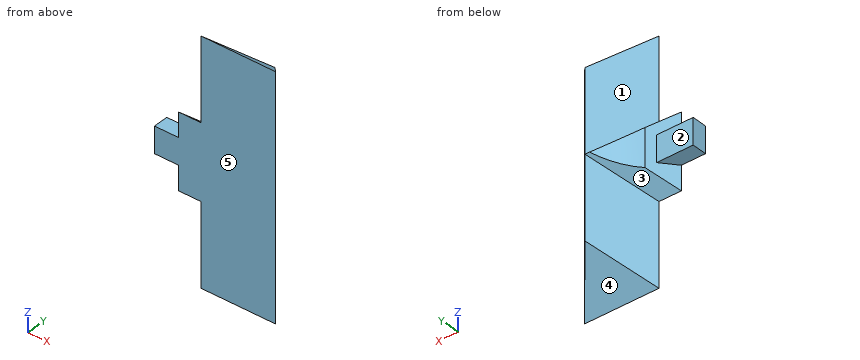
from build123d import *

# Parameters (mm, degrees)
BOSS_EXTRUDE1_START       = -105
BOSS_EXTRUDE1_DEPTH       = 160
BOSS_EXTRUDE1_2_DEPTH     = 40
BOSS_EXTRUDE1_START_2     = -20
BOSS_EXTRUDE1_3_OUTLINE_W = 47
BOSS_EXTRUDE1_3_OUTLINE_H = 147
BOSS_EXTRUDE1_3_DEPTH     = 20
BOSS_EXTRUDE1_START_3     = 42.132444372
BOSS_EXTRUDE1_4_OUTLINE_W = 53
BOSS_EXTRUDE1_4_OUTLINE_H = 116
BOSS_EXTRUDE1_4_DEPTH     = 19.867555628
BOSS_EXTRUDE1_START_4     = 80.434666527
BOSS_EXTRUDE1_5_OUTLINE_W = 52
BOSS_EXTRUDE1_5_OUTLINE_H = 117
BOSS_EXTRUDE1_5_DEPTH     = 20.565333473
SKETCH2_W                 = 32.400830654
SKETCH2_H                 = 17.550449938
BOSS_EXTRUDE2_DEPTH       = 10
SKETCH4_R                 = 75
CUT_EXTRUDE1_DEPTH        = 80


with BuildPart() as part:
    # Boss-Extrude1: read off the stored shape, not the designer's step
    # Boss-Extrude1 outline → Boss-Extrude1 (new body)
    with BuildSketch(Plane.XY.offset(BOSS_EXTRUDE1_START)):
        Polygon((65, 0), (40, 29.793839815), (15, 0), align=None)
    extrude(amount=BOSS_EXTRUDE1_DEPTH)

    # Boss-Extrude1 2 outline → Boss-Extrude1 2 (add)
    with BuildSketch(Plane.YZ):
        Polygon((0, -50), (29.793839815, -25), (0, 0), align=None)
    extrude(amount=BOSS_EXTRUDE1_2_DEPTH)

    # Boss-Extrude1 3 outline → Boss-Extrude1 3 (cut)
    with BuildSketch(Plane(origin=(0, 0, 0), x_dir=(0.6427876096865404, 0.7660444431189772, 0), z_dir=(0.7660444431189772, -0.6427876096865403, 0)).offset(BOSS_EXTRUDE1_START_2)):
        with Locations((22.5, -24.5)):
            Rectangle(BOSS_EXTRUDE1_3_OUTLINE_W, BOSS_EXTRUDE1_3_OUTLINE_H)
    extrude(amount=BOSS_EXTRUDE1_3_DEPTH, mode=Mode.SUBTRACT)

    # Boss-Extrude1 4 outline → Boss-Extrude1 4 (cut)
    with BuildSketch(Plane(origin=(0, 0, 0), x_dir=(1, 0, 0), z_dir=(0, 0.6427876096865403, 0.7660444431189772)).offset(BOSS_EXTRUDE1_START_3)):
        with Locations((40.5, 21)):
            Rectangle(BOSS_EXTRUDE1_4_OUTLINE_W, BOSS_EXTRUDE1_4_OUTLINE_H)
    extrude(amount=BOSS_EXTRUDE1_4_DEPTH, mode=Mode.SUBTRACT)

    # Boss-Extrude1 5 outline → Boss-Extrude1 5 (cut)
    with BuildSketch(Plane(origin=(0, 0, 0), x_dir=(1, 0, 0), z_dir=(0, 0.6427876096865403, -0.7660444431189772)).offset(BOSS_EXTRUDE1_START_4)):
        with Locations((40, 10.5)):
            Rectangle(BOSS_EXTRUDE1_5_OUTLINE_W, BOSS_EXTRUDE1_5_OUTLINE_H)
    extrude(amount=BOSS_EXTRUDE1_5_DEPTH, mode=Mode.SUBTRACT)

    # Sketch2 → Boss-Extrude2 (add)
    with BuildSketch(Plane.XZ):
        with Locations((0, -25)):
            Rectangle(SKETCH2_W, SKETCH2_H)
    extrude(amount=-BOSS_EXTRUDE2_DEPTH)

    # Sketch4 → Cut-Extrude1 (cut, symmetric)
    with BuildSketch(Plane.XY):
        with Locations((-13.767329279, 85)):
            Circle(SKETCH4_R)
    extrude(amount=CUT_EXTRUDE1_DEPTH, both=True, mode=Mode.SUBTRACT)


solid = part.part
Design review of the part built by this model. Coordinates are the model's own, in mm. Face numbers are marked on the shaded views. A direction names the side the tool comes from. Round coordinates to 2 decimals unless told otherwise and drop trailing zeros. Loops run counter-clockwise (first coordinate to the right, second up) from the corner with the lowest first, then second, coordinate; pieces in that order, holes last. Notation, with made-up numbers: M -35.75,-23 L -30.75,-23 A26 ccw -30.75,-8 Z; hole C 55,18 d2. An arc over 180 degrees is marked long. Answer as a JSON object with one key per item and string values.
Item 1: Clearance check with flat-ended pins moving along their axes: P1, Ø3, axis at y = 13, z = -66, coming from the -X side; P2, Ø8, axis at x = 33.5, z = -68.5, coming from the +Y side; P3, Ø11, axis at x = -2.5, y = 7, coming from the -Z side. State where each tip first meets the part, or that it passes through.
Answer sheet:
{"P1": "stops at x = 24.65", "P2": "stops at y = 26.81", "P3": "stops at z = -33.78"}
Item 2: We need section C-C on z = 24.5. Give the boundary of the cut face in (x, y), and give its area (3 significant figures).
Answer sheet:
{"outline": "M 15,0 L 65,0 L 40,29.79 Z", "area": "745 mm^2"}
Item 3: Wall thickness on L1, parallel to Z at x = 0, y = 8.5; L2, parallel to Y at x = 4.5, z = -27; L3, parallel to X at y = 12.5, z = -87.5: over which ranges is each line inside the solid? List them lowest first. Write a range as from..to.
Answer sheet:
{"L1": "z = -33.78..-16.22", "L2": "y = 0..10", "L3": "x = 25.49..54.51"}
Item 4: We need section A-A on x = 20.5. Give the boundary of the cut face in (y, z), and give its area (3 significant figures).
Answer sheet:
{"outline": "M 0,-105 L 6.55,-99.5 L 6.55,-44.5 L 18.29,-34.66 L 18.29,-15.34 L 6.55,-5.5 L 6.55,49.5 L 0,55 Z", "area": "1,350 mm^2"}
Item 5: Machinability: for the marked faces 1, 2, 3, 4 and 5, which of the approach directions +Z, -Z, +X, -X, +Y, -Y give a long, thin tool a straight path to every point of the face, cutting with its end or side? Answer none if there is none.
Answer sheet:
{"face 1": "+Z, -X, +Y", "face 2": "+Z, -Z, -X, +Y", "face 3": "-Z, -X, +Y", "face 4": "-Z, +X, -X, +Y", "face 5": "+Z, -Z, +X, -X, -Y"}
Item 6: We need section D-D on y = 3. Give the boundary of the cut face in (x, z).
Answer sheet:
{"outline": "M -16.2,-33.78 L 2.52,-33.78 L 2.52,-47.48 L 17.52,-47.48 L 17.52,-102.48 L 62.48,-102.48 L 62.48,52.48 L 17.52,52.48 L 17.52,-2.52 L 2.52,-2.52 L 2.52,-16.22 L -16.2,-16.22 Z"}
Item 7: We need section B-B on y = 22.25. Give the boundary of the cut face in (x, z).
Answer sheet:
{"outline": "M 27.31,-31.33 L 33.67,-31.33 L 33.67,-86.33 L 46.33,-86.33 L 46.33,36.33 L 33.67,36.33 L 33.67,-18.67 L 27.31,-18.67 Z"}
